Autodesk Inventor part; units mm, degrees
ref_plane "Work Plane1" through (0, -25.4, -12.4625) normal (0, 0, 1) x (1, 0, 0)
ref_plane "YZ Plane" through (0, 0, 0) normal (1, 0, 0) x (0, 1, 0)
ref_plane "XZ Plane" through (0, 0, 0) normal (0, 1, 0) x (-1, 0, 0)
sketch "Sketch1" plane through (0, 0, 0) normal (1, 0, 0) x (0, 1, 0)
  arc A0 (25.4, -19.293) -> (-25.4, -19.293) centre (0, -35.56) ccw
  line L0 (0, 0) -> (0, -134.2841)
  line L1 (-25.4, 0) -> (-25.4, -19.293)
  line L2 (25.4, -19.293) -> (25.4, 0)
  line L3 (25.4, 0) -> (25.4, 5)
  line L4 (25.4, 5) -> (-25.4, 5)
  line L5 (-25.4, 5) -> (-25.4, 0)
  dimension "d0" = 60.325
  dimension "d3" = 50.8
  dimension "d38" = 5
extrude "Extrusion1" add sketch "Sketch1" along normal blind 127
sketch "Sketch4" plane through (0, 25.4, 5) normal (0, 0, 1) x (1, 0, 0)
  circle A0 centre (25, -25.4) radius 13
  line L0 (0, 0) -> (127, 0)
  line L1 (0, 0) -> (0, -50.8)
  dimension "d20" = 26
  dimension "d39" = 25.4
  dimension "d40" = 25
extrude "Extrusion4" cut sketch "Sketch4" against normal through all
sketch "Sketch6" plane through (0, -25.4, 5) normal (0, 0, 1) x (1, 0, 0)
  line L0 (73.5, 38.1) -> (98.9, 38.1)
  line L1 (98.9, 38.1) -> (98.9, 12.7)
  line L2 (98.9, 12.7) -> (73.5, 12.7)
  line L3 (73.5, 12.7) -> (73.5, 38.1)
  line L4 (0, 0) -> (127, 0) construction
  line L5 (0, 50.8) -> (127, 50.8)
  line L6 (0, 50.8) -> (0, 0)
  point P0 (0, 25.4)
  point P1 (73.5, 25.4)
  dimension "d35" = 25.4
  dimension "d36" = 25.4
  dimension "d41" = 25.4
  dimension "d42" = 73.5
hole "Hole1" at (73.5, 12.7, 5) at (98.9, 12.7, 5) at (98.9, -12.7, 5) at (73.5, -12.7, 5) direction (0, 0, -1) diameter 6.756 end through all
ref_plane "Work Plane1" through (0, -25.4, -12.4625) normal (0, 0, 1) x (1, 0, 0)
sketch "Sketch7" plane through (0, -25.4, -12.4625) normal (0, 0, 1) x (1, 0, 0)
  circle A0 centre (73.5, 38.1) radius 3.378
  circle A1 centre (73.5, 38.1) radius 5.08
  circle A2 centre (73.5, 12.7) radius 3.378
  circle A3 centre (73.5, 12.7) radius 5.08
  circle A4 centre (98.9, 12.7) radius 3.378
  circle A5 centre (98.9, 12.7) radius 5.08
  circle A6 centre (98.9, 38.1) radius 3.378
  circle A7 centre (98.9, 38.1) radius 5.08
  point P0 (0, 25.4)
  dimension "d44" = 10.16
extrude "Extrusion5" cut sketch "Sketch7" along normal blind 10 contours A0 | A1 | A2 | A3 | A4 | A5 | A6 | A7
properties part number "Motor Mount" material "ABS Plastic"
Could you check a few things on this model? Use its own coordinates, in mm. A direction names the side the tool comes from. Give positions to 0.01 mm unless a question says otherwise; leave off trailing zeros. Order: outer loops, then holes, each group sorted by start corner. A loop starts at its lowest first (then second) coordinate and runs counter-clockwise, first axis right, second up. Notation, with made-up numbers: (68, 13) - (85, 13) arc R23 ccw to (85, 49) - close; hole circle Ø9 at (-6, 43). An arc over 180 degrees is marked (long way). Return JSON: item names as keys, results as strings. Group by question number.
Q1. Suppose I cut it at C-C, the plane z = -3.75. Please give me the cut outline in (x, y).
Q2. Will these pins go through, and if not, where does the flat tip stop? pin 1 Ø16.5 at (x, y) = (98.9, -12.7) entering from -Z; pin 2 Ø5.5 at (x, y) = (98.9, 12.7) entering from +Z; pin 3 Ø8 at (x, y) = (99.5, 12) entering from -Z; pin 4 Ø8 at (x, y) = (72, -14.5) entering from -Z.
Q3. Suppose I cut it at A-A, the plane y = 0. Please give me the cut outline in (x, z), and give its area (3 significant figures).
Q4. Suppose I cut it at D-D, the plane x = 72. Please give me the cut outline in (y, z), and give its area (3 significant figures).
Q5. Which directions (+Z, -Z, +X, -X, +Y, -Y) give clear straight access to the entire face, cutting with the end or side of a thin tool? Please do faces 4 (the face through (98.239, -17.737, -5.92)), 5 (the face through (0, 0, -2)).
Q6. Thinking about a two-plate mould opening in X: for faces 1 (the face through (127, 0, -2)), 2 (the face through (63, 25.4, -7)), 3 (the face through (77, -14, -2.462)), which applies, pulls with the +X half, pulls with the -X half, needs draft (parallel to the pull), parting line crosses it, or undercut?
Q7. Please list where these lines run through material, in increasing order: line 1 along Y through (x, z) = (98.9, 0); line 2 along Y through (x, z) = (73.5, -8.75); line 3 along X through (y, z) = (-9, -2.5). Write a range as [from, to].
Q8. Suppose I cut it at B-B, the plane x = 25. Please give me the cut outline in (y, z).
Resolved:
{
 "1": {"outline": "(0, -25.4) - (127, -25.4) - (127, 25.4) - (0, 25.4) - close; hole circle Ø26 at (25, 0); hole circle Ø10.16 at (73.5, -12.7); hole circle Ø10.16 at (73.5, 12.7); hole circle Ø10.16 at (98.9, -12.7); hole circle Ø10.16 at (98.9, 12.7)"},
 "2": {"pin 1": "stops at z = -13.86", "pin 2": "passes through", "pin 3": "stops at z = -2.46", "pin 4": "stops at z = -11.74"},
 "3": {"outline": "(0, -5.4) - (12, -5.4) - (12, 5) - (0, 5) - close; (38, -5.4) - (127, -5.4) - (127, 5) - (38, 5) - close", "area": "1,050 mm2"},
 "4": {"outline": "(-25.4, -19.29) arc R30.16 cw to (-17.55, -11.03) - (-17.55, -2.46) - (-15.73, -2.46) - (-15.73, 5) - (-25.4, 5) - close; (-9.67, -2.46) - (-7.85, -2.46) - (-7.85, -6.44) arc R30.16 cw to (7.85, -6.44) - (7.85, -2.46) - (9.67, -2.46) - (9.67, 5) - (-9.67, 5) - close; (15.73, -2.46) - (17.55, -2.46) - (17.55, -11.03) arc R30.16 cw to (25.4, -19.29) - (25.4, 5) - (15.73, 5) - close", "area": "531 mm2"},
 "5": {"face 4": "-Z", "face 5": "+Z, -Z, -X, +Y, -Y"},
 "6": {"face 1": "pulls with the +X half", "face 2": "needs draft", "face 3": "undercut"},
 "7": {"line 1": "y = [-25.4, -16.08], [-9.32, 9.32], [16.08, 25.4]", "line 2": "y = [-25.4, -17.78], [17.78, 25.4]", "line 3": "x = [0, 15.62], [34.38, 70.02], [76.98, 95.42], [102.38, 127]"},
 "8": {"outline": "(-25.4, -19.29) arc R30.16 cw to (-13, -8.34) - (-13, 5) - (-25.4, 5) - close; (13, -8.34) arc R30.16 cw to (25.4, -19.29) - (25.4, 5) - (13, 5) - close"}
}
